Input: part model. Units: mm. Frame: model coordinates. Round coordinates to 2 decimals unless told otherwise and drop trailing zeros. Loops run counter-clockwise (first coordinate to the right, second up) from the corner with the lowest first, then second, coordinate; pieces in that order, holes last. Notation, with made-up numbers: (-21, 56) - (-9, 56) arc R14 cw to (-9, 78) - close; hole circle Ø2 at (33, 48.25). An arc over 180 degrees is marked (long way). One line per question, with ' | ' between items. Start each with the question number.
Item 1: Section A-A, the plane y = 1. Return loops of the section in (x, z), plus the area to 3 significant figures.
Item 2: Section C-C, the plane z = -90. Return loops of the section in (x, y), plus the area to 3 significant figures.
Item 3: Material intervals for line 1 along Z through (x, y) = (-44, 4.25); line 2 along X through (y, z) = (2.25, -114), sorted ascending.
Item 4: Section B-B, the plane x = -39. Return loops of the section in (y, z), plus the area to 3 significant figures.
```python
from build123d import *

# Parameters (mm, degrees)
SKETCH1_W           = 53.594
SKETCH1_H           = 82.55
BOSS_EXTRUDE1_DEPTH = 6.35
SKETCH6_W           = 53.594
SKETCH6_H           = 6.35
BOSS_EXTRUDE3_DEPTH = 7.62
SKETCH3_W           = 0.508
SKETCH3_H           = 90.17
CUT_EXTRUDE2_DEPTH  = 6.35
SKETCH8_W           = 37.338
SKETCH8_H           = 6.35
BOSS_EXTRUDE4_DEPTH = 43.18
SKETCH10_W          = 53.153164817
SKETCH10_H          = 6.35
BOSS_EXTRUDE5_DEPTH = 90.17
SKETCH11_W          = 0.575164817
SKETCH11_H          = 6.35
BOSS_EXTRUDE6_DEPTH = 43.18


with BuildPart() as part:
    # Sketch1 → Boss-Extrude1 (new body)
    with BuildSketch(Plane(origin=(0, 0, 0), x_dir=(1, 0, 0), z_dir=(0, 1, 0))):
        with Locations((-26.797, 41.275)):
            Rectangle(SKETCH1_W, SKETCH1_H)
    extrude(amount=BOSS_EXTRUDE1_DEPTH)

    # Sketch6 → Boss-Extrude3 (add)
    with BuildSketch(Plane.XY):
        with Locations((-26.797, 3.175)):
            Rectangle(SKETCH6_W, SKETCH6_H)
    extrude(amount=BOSS_EXTRUDE3_DEPTH)

    # Sketch3 → Cut-Extrude2 (cut)
    with BuildSketch(Plane(origin=(0, 6.35, 0), x_dir=(1, 0, 0), z_dir=(0, 1, 0))):
        with Locations((-0.254, 37.465)):
            Rectangle(SKETCH3_W, SKETCH3_H)
    cut_extrude2 = extrude(amount=-CUT_EXTRUDE2_DEPTH, mode=Mode.SUBTRACT)

    # Mirror1: Cut-Extrude2 across plane
    add(cut_extrude2.mirror(Plane(origin=(-26.797, 0, 0), x_dir=(0, 0, 1), z_dir=(1, 0, 0))), mode=Mode.SUBTRACT)

    # Sketch8 → Boss-Extrude4 (add)
    with BuildSketch(Plane(origin=(0, 0, -82.55), x_dir=(-1, 0, 0), z_dir=(0, 0, -1))):
        with Locations((19.177, 3.175)):
            Rectangle(SKETCH8_W, SKETCH8_H)
    extrude(amount=BOSS_EXTRUDE4_DEPTH)

    # Sketch10 → Boss-Extrude5 (add)
    with BuildSketch(Plane.XY.offset(7.62)):
        with Locations((-26.509417592, 3.175)):
            Rectangle(SKETCH10_W, SKETCH10_H)
    extrude(amount=-BOSS_EXTRUDE5_DEPTH)

    # Sketch11 → Boss-Extrude6 (add)
    with BuildSketch(Plane(origin=(0, 0, -82.55), x_dir=(-1, 0, 0), z_dir=(0, 0, -1))):
        with Locations((0.220417592, 3.175)):
            Rectangle(SKETCH11_W, SKETCH11_H)
    extrude(amount=BOSS_EXTRUDE6_DEPTH)


solid = part.part
```
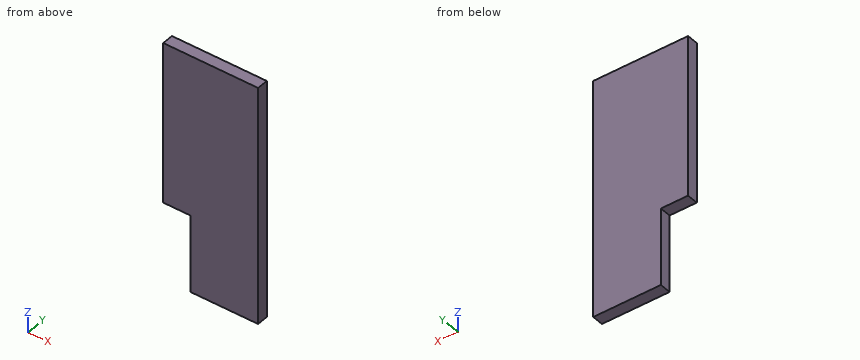
Return value:
1) outline: (-53.09, -82.55) - (-37.85, -82.55) - (-37.85, -125.73) - (0.07, -125.73) - (0.07, 7.62) - (-53.09, 7.62) - close | area: 6,430 mm2
2) outline: (-37.85, 0) - (0.07, 0) - (0.07, 6.35) - (-37.85, 6.35) - close | area: 241 mm2
3) line 1: -82.55 to 7.62 | line 2: -37.85 to 0.07
4) outline: (0, -82.55) - (6.35, -82.55) - (6.35, 7.62) - (0, 7.62) - close | area: 573 mm2
